Part model, mm, in its own coordinate system. Give positions to 0.01 mm unless a question says otherwise; leave off trailing zeros. Order: outer loops, then holes, each group sorted by start corner. A loop starts at its lowest first (then second) coordinate and runs counter-clockwise, first axis right, second up. Notation, with made-up numbers: M 56,24 L 68,24 A16 ccw 68,48 Z; hole C 16,-6.75 d8. An arc over 180 degrees is marked long. Return JSON: item names as keys, results as strings.
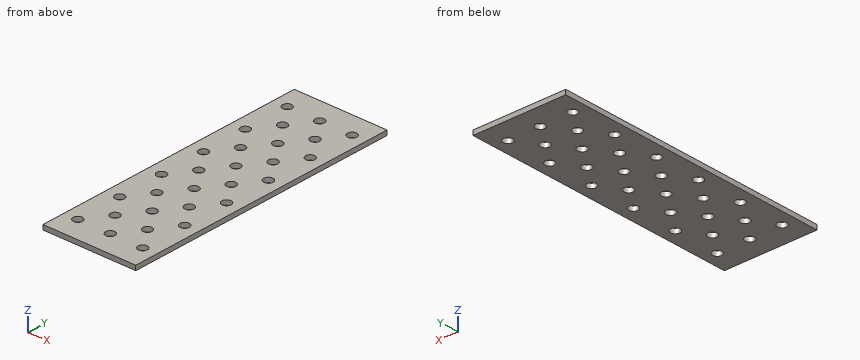
from build123d import *

# Parameters (mm, degrees)
SKETCH1_W          = 40
SKETCH1_H          = 120
SKETCH1_R          = 2
BASE_FLANGE1_DEPTH = 2


# Sheet-metal steps are written as plain solids
with BuildPart() as part:
    # Sketch1 → Base-Flange1 (new body)
    with BuildSketch(Plane.XY):
        Rectangle(SKETCH1_W, SKETCH1_H)
        with Locations((-14, 50)):
            Circle(SKETCH1_R, mode=Mode.SUBTRACT)
        with Locations((0, 50)):
            Circle(SKETCH1_R, mode=Mode.SUBTRACT)
        with Locations((14, 50)):
            Circle(SKETCH1_R, mode=Mode.SUBTRACT)
        with Locations((-7, 40)):
            Circle(SKETCH1_R, mode=Mode.SUBTRACT)
        with Locations((7, 40)):
            Circle(SKETCH1_R, mode=Mode.SUBTRACT)
        with Locations((-14, 30)):
            Circle(SKETCH1_R, mode=Mode.SUBTRACT)
        with Locations((-7, 20)):
            Circle(SKETCH1_R, mode=Mode.SUBTRACT)
        with Locations((7, 20)):
            Circle(SKETCH1_R, mode=Mode.SUBTRACT)
        with Locations((0, 30)):
            Circle(SKETCH1_R, mode=Mode.SUBTRACT)
        with Locations((14, 30)):
            Circle(SKETCH1_R, mode=Mode.SUBTRACT)
        with Locations((-14, 10)):
            Circle(SKETCH1_R, mode=Mode.SUBTRACT)
        with Locations((-7, 0)):
            Circle(SKETCH1_R, mode=Mode.SUBTRACT)
        with Locations((7, 0)):
            Circle(SKETCH1_R, mode=Mode.SUBTRACT)
        with Locations((0, 10)):
            Circle(SKETCH1_R, mode=Mode.SUBTRACT)
        with Locations((14, 10)):
            Circle(SKETCH1_R, mode=Mode.SUBTRACT)
        with Locations((-14, -10)):
            Circle(SKETCH1_R, mode=Mode.SUBTRACT)
        with Locations((-7, -20)):
            Circle(SKETCH1_R, mode=Mode.SUBTRACT)
        with Locations((7, -20)):
            Circle(SKETCH1_R, mode=Mode.SUBTRACT)
        with Locations((0, -10)):
            Circle(SKETCH1_R, mode=Mode.SUBTRACT)
        with Locations((14, -10)):
            Circle(SKETCH1_R, mode=Mode.SUBTRACT)
        with Locations((-14, -30)):
            Circle(SKETCH1_R, mode=Mode.SUBTRACT)
        with Locations((-7, -40)):
            Circle(SKETCH1_R, mode=Mode.SUBTRACT)
        with Locations((7, -40)):
            Circle(SKETCH1_R, mode=Mode.SUBTRACT)
        with Locations((0, -30)):
            Circle(SKETCH1_R, mode=Mode.SUBTRACT)
        with Locations((14, -30)):
            Circle(SKETCH1_R, mode=Mode.SUBTRACT)
        with Locations((-14, -50)):
            Circle(SKETCH1_R, mode=Mode.SUBTRACT)
        with Locations((0, -50)):
            Circle(SKETCH1_R, mode=Mode.SUBTRACT)
        with Locations((14, -50)):
            Circle(SKETCH1_R, mode=Mode.SUBTRACT)
    extrude(amount=-BASE_FLANGE1_DEPTH)


solid = part.part
Q1. Probe line 1 along Y through (x, z) = (-7, -0.85); line 2 along X through (y, z) = (-51, -0.9); line 3 along X through (y, z) = (-28.5, -1.65). List the from-to ranges inside material, lowest first.
Established:
{"line 1": "y = -60 to -42, -38 to -22, -18 to -2, 2 to 18, 22 to 38, 42 to 60", "line 2": "x = -20 to -15.73, -12.27 to -1.73, 1.73 to 12.27, 15.73 to 20", "line 3": "x = -20 to -15.32, -12.68 to -1.32, 1.32 to 12.68, 15.32 to 20"}
Q2. Pin check, flat tips, straight feed: pin 1 (6.5 mm diameter, centred on x = 14, y = -10, fed in from +Z); pin 2 (3 mm diameter, centred on x = 14, y = -30, fed in from -Z). Stop position of each tip, or through.
Established:
{"pin 1": "stops at z = 0", "pin 2": "passes through"}
Q3. Band-saw the part on A-A (y = -30). Give the cut face in (x, z), then the cut area to 3 significant figures.
Established:
{"outline": "M -20,-2 L -16,-2 L -16,0 L -20,0 Z; M -12,-2 L -2,-2 L -2,0 L -12,0 Z; M 2,-2 L 12,-2 L 12,0 L 2,0 Z; M 16,-2 L 20,-2 L 20,0 L 16,0 Z", "area": "56.0 mm²"}
Q4. Band-saw the part on C-C (y = 40). Give the cut face in (x, z).
Established:
{"outline": "M -20,-2 L -9,-2 L -9,0 L -20,0 Z; M -5,-2 L 5,-2 L 5,0 L -5,0 Z; M 9,-2 L 20,-2 L 20,0 L 9,0 Z"}
Q5. Band-saw the part on B-B (x = -14). Give the cut face in (y, z).
Established:
{"outline": "M -60,-2 L -52,-2 L -52,0 L -60,0 Z; M -48,-2 L -32,-2 L -32,0 L -48,0 Z; M -28,-2 L -12,-2 L -12,0 L -28,0 Z; M -8,-2 L 8,-2 L 8,0 L -8,0 Z; M 12,-2 L 28,-2 L 28,0 L 12,0 Z; M 32,-2 L 48,-2 L 48,0 L 32,0 Z; M 52,-2 L 60,-2 L 60,0 L 52,0 Z"}
Q6. Band-saw the part on D-D (z = -1.15). Give the number of separate pieces and of enclosed holes in the cut face, then the cut area to 3 significant figures.
Established:
{"separate pieces": "1", "enclosed holes": "28", "area": "4,450 mm²"}
